Here's the drawing with two shaded views (mm, measured from the low corner). I have some questions. Round coordinates to 2 decimals unless told otherwise and drop trailing zeros. Loops run counter-clockwise (first coordinate to the right, second up) from the corner with the lowest first, then second, coordinate; pieces in that order, holes last. Notation, with made-up numbers: (68, -19) -> (122, -19) arc R23 ccw to (122, 18) -> close; hole circle Ø4 at (77, -10). An arc over 180 degrees is marked (long way). Write item = value, one per line.
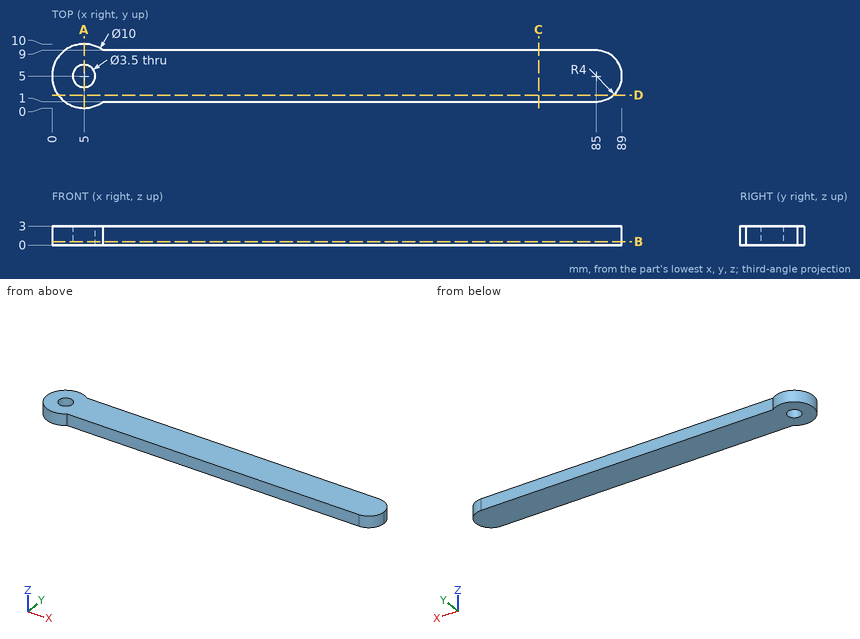
1. I need wall thicknesses on line 1 (Y direction, x = 5, z = 2.15); line 2 (Y direction, x = 12, z = 2.2); line 3 (X direction, y = 4.25, z = 2.1). Which ranges of each line are inside material? Lowest first, please. Write a range as [from, to].
Entries:
line_1 = [0, 3.25], [6.75, 10]
line_2 = [1, 9]
line_3 = [0.06, 3.42], [6.58, 88.93]
2. Suppose I cut it at C-C, the plane x = 76. List the corners of the cut face in (y, z) for me.
Entries:
outline = (1, 0) -> (9, 0) -> (9, 3) -> (1, 3) -> close
3. Suppose I cut it at A-A, the plane x = 5. List the corners of the cut face in (y, z) for me.
Entries:
outline = (0, 0) -> (3.25, 0) -> (3.25, 3) -> (0, 3) -> close; (6.75, 0) -> (10, 0) -> (10, 3) -> (6.75, 3) -> close
4. Suppose I cut it at B-B, the plane z = 0.55. List the corners of the cut face in (x, y) for me, and give its area (3 significant figures).
Entries:
outline = (8, 1) -> (85, 1) arc R4 ccw to (85, 9) -> (8, 9) arc R5 ccw (long way) to start; hole circle Ø3.5 at (5, 5)
area = 699 mm²
5. Suppose I cut it at D-D, the plane y = 2. List the corners of the cut face in (x, z) for me, and give its area (3 significant figures).
Entries:
outline = (1, 0) -> (87.65, 0) -> (87.65, 3) -> (1, 3) -> close
area = 260 mm²
6. I'm going to push flat-ended pins straight in: pin 1 (2 mm diameter, centred on x = 5, y = 5, fed in from -Z); pin 2 (1 mm diameter, centred on x = 73, z = 0.5, fed in from -Y). Where does each tip first touch, or does it pass through?
Entries:
pin_1 = through
pin_2 = 1
